Work out the finished part from the listing and answer in its coordinate system (mm). Face numbers are marked on the shaded views. A direction names the side the tool comes from. Round coordinates to 2 decimals unless told otherwise and drop trailing zeros. Loops run counter-clockwise (first coordinate to the right, second up) from the corner with the lowest first, then second, coordinate; pieces in that order, holes last. Notation, with made-up numbers: M 40,-37 L 50,-37 A10 cw 50,-18 Z; hole C 9.5,30.5 d11. An arc over 180 degrees is marked long. One line per item, written item: value.
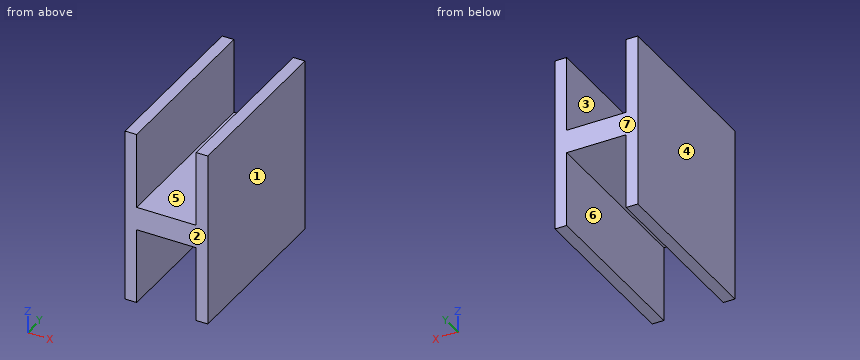
```python
from build123d import *

# Parameters (mm, degrees)
F1_DEPTH = 30


with BuildPart() as f1:
    # F0 (on Front) → F1 (new body)
    with BuildSketch(Plane.XZ):
        Polygon((-7.1, 2), (-7.1, 0), (7.1, 0), (7.1, 2), (7.1, 15), (5.1, 15), (5.1, 2), (-5.1, 2), (-5.1, 15), (-7.1, 15), align=None)
    extrude(amount=-F1_DEPTH)

    # F2: F1 across face


with BuildPart() as f1_1:
    add(f1.part)
    add(f1.part.mirror(Plane(origin=(0, 15, 0), x_dir=(1, 0, 0), z_dir=(0, 0, -1))))


solid = f1_1.part
```
1) The mould has two halves that part along X. Classify the marked faces 1, 2, 3 and 4: +X half, -X half, draft (parallel to the pull), parting line (faces both ways), or undercut.
Check values:
face 1: +X half
face 2: draft
face 3: undercut
face 4: -X half
2) For the marked faces 5, 6 and 7, determine the directions among +Z, -Z, +X, -X, +Y, -Y from which every point of the face is accessible in a straight line to the end or side of a thin tool.
Check values:
face 5: +Z, +Y, -Y
face 6: -Z, +Y, -Y
face 7: +Z, -Z, +X, -X, +Y
3) Find section A-A (z = 11). Give the vertices of the cut face in (x, y), then the cut area to 3 significant figures.
Check values:
outline: M -7.1,0 L -5.1,0 L -5.1,30 L -7.1,30 Z; M 5.1,0 L 7.1,0 L 7.1,30 L 5.1,30 Z
area: 120 mm2
4) Find section B-B (y = 22.25). Give the vertices of the cut face in (x, z), then the cut area to 3 significant figures.
Check values:
outline: M -7.1,-15 L -5.1,-15 L -5.1,-2 L 5.1,-2 L 5.1,-15 L 7.1,-15 L 7.1,15 L 5.1,15 L 5.1,2 L -5.1,2 L -5.1,15 L -7.1,15 Z
area: 161 mm2
5) This flat-tipped pin is pushed along its axis until it touches: pin 1 (3 mm diameter, centred on x = -1, y = 9.5, fed in from -Z). Where does it stop, or does it pass through?
Check values:
pin 1: z = -2
6) Find the intervals of material crossed by probe 1 along X at (y, z) = (28, -8); probe 2 along Z at (x, y) = (4, 22.5), in increasing order. Write a range as from..to.
Check values:
probe 1: -7.1..-5.1, 5.1..7.1
probe 2: -2..2
7) Find section C-C (x = 3.5). Give the vertices of the cut face in (y, z), then the cut area to 3 significant figures.
Check values:
outline: M 0,-2 L 30,-2 L 30,2 L 0,2 Z
area: 120 mm2
